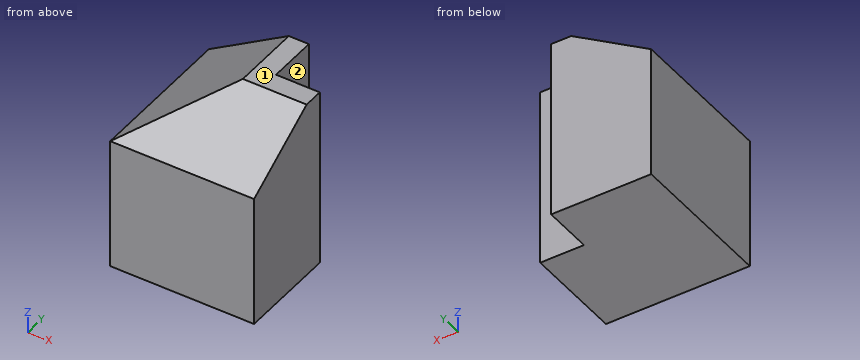
from build123d import *

# Parameters (mm, degrees)
PAD014_DEPTH    = 28.8
POCKET011_DEPTH = 24
POCKET012_DEPTH = 24
SKETCH112_W     = 1
SKETCH112_H     = 16
POCKET028_DEPTH = 30
PAD141_DEPTH    = 23
PAD142_DEPTH    = 24
POCKET056_DEPTH = 24
POCKET057_DEPTH = 23


with BuildPart() as part:
    # Sketch025 (on Face52 of Binder010) → Pad014 (new body)
    with BuildSketch(Plane.XY.offset(-28.8)):
        Polygon((0, 0), (0, 8), (-16, 8), (-16, -16), (8, -16), (8, 0), align=None)
    extrude(amount=PAD014_DEPTH)

    # Sketch026 (on Face5 of Pad014) → Pocket011 (cut)
    with BuildSketch(Plane.YZ.offset(8)):
        Polygon((-16, -9.6), (0, 0), (-16, 0), align=None)
    extrude(amount=-POCKET011_DEPTH, mode=Mode.SUBTRACT)

    # Sketch027 (on Face3 of Pocket011) → Pocket012 (cut)
    with BuildSketch(Plane(origin=(0, 8, 0), x_dir=(-1, 0, 0), z_dir=(0, 1, 0))):
        Polygon((16, -9.6), (0, 0), (16, 0), align=None)
    extrude(amount=-POCKET012_DEPTH, mode=Mode.SUBTRACT)

    # Sketch112 (on Face4 of Pocket012) → Pocket028 (cut)
    with BuildSketch(Plane(origin=(0, 0, -28.8), x_dir=(1, 0, 0), z_dir=(0, 0, -1))):
        with Locations((7.5, 8)):
            Rectangle(SKETCH112_W, SKETCH112_H)
    extrude(amount=-POCKET028_DEPTH, mode=Mode.SUBTRACT)

    # Sketch137 (on Face7 of Pocket028) → Pad141 (join)
    with BuildSketch(Plane.YZ.offset(7)):
        Polygon((0, 0), (-3.2, 0), (-16, -7.68), (-16, -10.88), (-3.2, -3.2), (0, -3.2), align=None)
    extrude(amount=-PAD141_DEPTH)

    # Sketch167 → Pad142 (join)
    with BuildSketch(Plane(origin=(0, 8, 0), x_dir=(-1, 0, 0), z_dir=(0, 1, 0))):
        Polygon((0, 0), (0, -3.2), (3.2, -3.2), (16, -10.88), (16, -7.68), (3.2, 0), align=None)
    extrude(amount=-PAD142_DEPTH)

    # Sketch170 (on Face9 of Pad142) → Pocket056 (cut)
    with BuildSketch(Plane(origin=(0, 8, 0), x_dir=(-1, 0, 0), z_dir=(0, 1, 0))):
        Polygon((3.2, 0), (16, -7.68), (16, 0), align=None)
    extrude(amount=-POCKET056_DEPTH, mode=Mode.SUBTRACT)

    # Sketch171 (on Face3 of Pocket056) → Pocket057 (cut)
    with BuildSketch(Plane.YZ.offset(7)):
        Polygon((-3.2, 0), (-16, -7.68), (-16, 0), align=None)
    extrude(amount=-POCKET057_DEPTH, mode=Mode.SUBTRACT)


solid = part.part
Can you work these out from the model? Positions are in its coordinate system, mm. Face numbers are marked on the shaded views. A direction names the side the tool comes from. Round coordinates to 2 decimals unless told otherwise and drop trailing zeros. Loops run counter-clockwise (first coordinate to the right, second up) from the corner with the lowest first, then second, coordinate; pieces in that order, holes last. Notation, with made-up numbers: (-27, 44.5) - (29, 44.5) arc R19 ccw to (29, 75.5) - close; hole circle Ø11 at (54, 35). An arc over 180 degrees is marked (long way). Use CSV: the item, a comma, the result in double quotes. Start each with the question number.
1) If we section it at B-B on x = 4.5: Write out the boundary of the cut face in (y, z), plus the area to 3 significant figures.
2) Please list where these lines run through material, in increasing order: probe 1 along Y at (x, z) = (1.5, -7.75); probe 2 along X at (y, z) = (-10.75, -5.75). Write a range as [from, to].
3) For the marked faces 1 and 2, which set-ups out of +Z, -Z, +X, -X, +Y, -Y let a thin tool reach every point of the face, with its end or its side?
4) For pin 1 Ø4 at (y, z) = (6, -13) entering from +X; pin 2 Ø6 at (x, y) = (-3.5, -7) entering from +Z; pin 3 Ø8 at (x, y) = (-9, -6) entering from +Z, each with a flat end and sliding along its axis, tell me the tip position at first contact or that it passes through.
5) If we section it at C-C on z = -11.25: Write out the boundary of the cut face in (x, y), plus the area to 3 significant figures.
6) If we section it at A-A on y = -11.5: Write out the boundary of the cut face in (x, z), plus the area to 3 significant figures.
Geometry results:
1,outline,"(-16, -28.8) - (0, -28.8) - (0, 0) - (-3.2, 0) - (-16, -7.68) - close"
1,area,"412 mm2"
2,probe 1,"y = [-16, 0]"
2,probe 2,"x = [-12.78, 7]"
3,face 1,"+Z, +X, -X, +Y, -Y"
3,face 2,"+Z, -Z, +X, +Y"
4,pin 1,"stops at x = 0"
4,pin 2,"stops at z = -0.48"
4,pin 3,"stops at z = -1.14"
5,outline,"(-16, -16) - (7, -16) - (7, 0) - (0, 0) - (0, 8) - (-16, 8) - close"
5,area,"496 mm2"
6,outline,"(-16, -28.8) - (7, -28.8) - (7, -4.98) - (-11.5, -4.98) - (-16, -7.68) - close"
6,area,"542 mm2"
